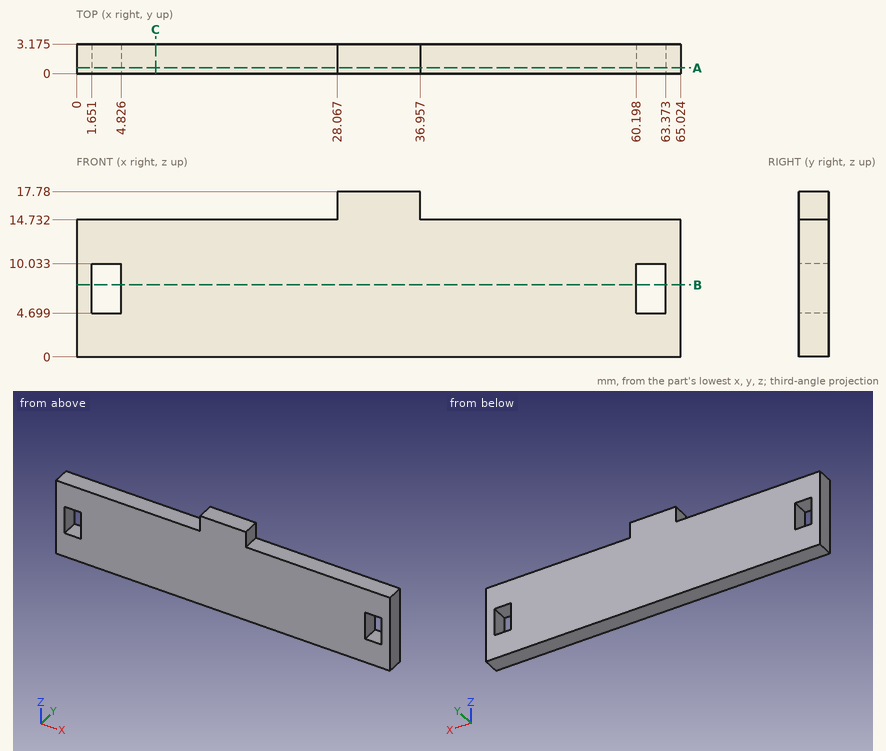
Source: three-view drawing plus pictorial views. Frame: mm from the lowest corner of the part. Coordinates: 2 decimals unless noted, no trailing zeros. Loops run counter-clockwise (first coordinate to the right, second up) from the corner with the lowest first, then second, coordinate; pieces in that order, holes last. Notation, with made-up numbers: (77.25, 35) - (114.25, 35) arc R23 ccw to (114.25, 65) - close; hole circle Ø5 at (-29.5, -23). An arc over 180 degrees is marked (long way). One line per item, written item: value. Start each with the question number.
1. Contact query for flat-ended pins moving along their axis: P1, Ø3, axis at x = 13.5, z = 10, coming from the -Y side; P2, Ø1.5, axis at y = 2, z = 16, coming from the +X side; P3, Ø1.5, axis at y = 1, z = 17, coming from the -X side. Output: stop coordinate, or through.
2. Section B-B (z = 7.75). Return the cut outline in (x, y) (3 decimals).
3. Ray query, L1, parallel to X at y = 2.65, z = 5.75; L2, parallel to Z at x = 61, y = 2; L3, parallel to Z at x = 53, y = 3. Return the intervals inside material, ascending.
4. Section C-C (x = 8.5). Return the cut outline in (y, z) (3 decimals).
5. Section A-A (y = 0.6). Return the cut outline in (x, z), and give its area (3 significant figures).
Verdict:
1. P1: stops at y = 0
1. P2: stops at x = 36.96
1. P3: stops at x = 28.07
2. outline: (0, 0) - (1.651, 0) - (1.651, 3.175) - (0, 3.175) - close; (4.826, 0) - (60.198, 0) - (60.198, 3.175) - (4.826, 3.175) - close; (63.373, 0) - (65.024, 0) - (65.024, 3.175) - (63.373, 3.175) - close
3. L1: x = 0 to 1.65, 4.83 to 60.2, 63.37 to 65.02
3. L2: z = 0 to 4.7, 10.03 to 14.73
3. L3: z = 0 to 14.73
4. outline: (0, 0) - (3.175, 0) - (3.175, 14.732) - (0, 14.732) - close
5. outline: (0, 0) - (65.02, 0) - (65.02, 14.73) - (36.96, 14.73) - (36.96, 17.78) - (28.07, 17.78) - (28.07, 14.73) - (0, 14.73) - close; hole (1.65, 4.7) - (4.83, 4.7) - (4.83, 10.03) - (1.65, 10.03) - close; hole (60.2, 4.7) - (63.37, 4.7) - (63.37, 10.03) - (60.2, 10.03) - close
5. area: 951 mm2
